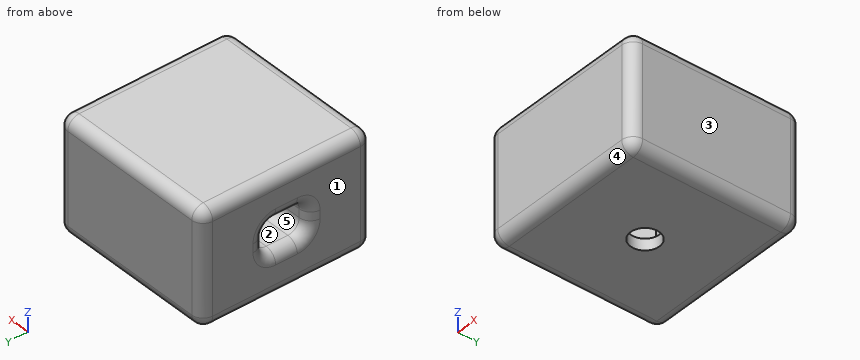
```python
from build123d import *

# Parameters (mm, degrees)
F0_W      = 38.1
F0_H      = 38.1
F1_DEPTH  = 25.4
F2_R      = 2.54
F4_DEPTH  = 33.02
F6_DEPTH  = 6.096
F7_DEPTH  = 2.54
F8_R      = 2.54
F9_R      = 3.211175
F10_DEPTH = 5.08


with BuildPart() as f1:
    # F0 (on Top) → F1 (new body)
    with BuildSketch(Plane.XY):
        Rectangle(F0_W, F0_H)
    extrude(amount=F1_DEPTH)

    # F2
    f2_edges = [f1.edges().sort_by_distance(p)[0] for p in [
        (-19.05, -19.05, 12.7),
        (-19.05, 0, 0),
        (19.05, -19.05, 12.7),
        (0, -19.05, 0),
        (0, -19.05, 25.4),
        (19.05, 0, 0),
        (0, 19.05, 0),
        (-19.05, 19.05, 12.7),
        (-19.05, 0, 25.4),
        (19.05, 0, 25.4),
        (0, 19.05, 25.4),
        (19.05, 19.05, 12.7),
    ]]
    fillet(f2_edges, radius=F2_R)

    # F3 (on face) → F4 (cut)
    with BuildSketch(Plane(origin=(-19.05, 0, 0), x_dir=(0, -1, 0), z_dir=(-1, 0, 0))):
        Polygon((4.958837, 16.184959), (0, 16.184959), (0, 12.7), (0, 9.215041), (4.958837, 9.215041), align=None)
        Polygon((0, 16.184959), (-4.958837, 16.184959), (-4.958837, 9.215041), (0, 9.215041), (0, 12.7), align=None)
    extrude(amount=-F4_DEPTH, mode=Mode.SUBTRACT)

    # F5 (on face) → F6 (cut)
    with BuildSketch(Plane(origin=(0, 0, 0), x_dir=(1, 0, 0), z_dir=(0, 0, -1))):
        Polygon((-2.712969, -4.699), (2.712969, -4.699), (5.425938, 0), (2.712969, 4.699), (-2.712969, 4.699), (-5.425938, 0), align=None)
    extrude(amount=-F6_DEPTH, mode=Mode.SUBTRACT)

    # F5 (on face) → F7 (join)
    with BuildSketch(Plane(origin=(0, 0, 0), x_dir=(1, 0, 0), z_dir=(0, 0, -1))):
        Polygon((-2.712969, -4.699), (2.712969, -4.699), (5.425938, 0), (2.712969, 4.699), (-2.712969, 4.699), (-5.425938, 0), align=None)
    extrude(amount=-F7_DEPTH)

    # F8
    f8_edges = [f1.edges().sort_by_distance(p)[0] for p in [
        (13.97, 0, 16.184959),
        (13.97, 4.958837, 12.7),
        (13.97, 0, 9.215041),
        (13.97, -4.958837, 12.7),
        (-2.54, 4.958837, 16.184959),
        (-2.54, 4.958837, 9.215041),
        (-19.05, 4.958837, 12.7),
        (-2.54, -4.958837, 16.184959),
        (-19.05, 0, 16.184959),
        (-2.54, -4.958837, 9.215041),
        (-19.05, -4.958837, 12.7),
        (-19.05, 0, 9.215041),
    ]]
    fillet(f8_edges, radius=F8_R)

    # F9 (on face) → F10 (cut)
    with BuildSketch(Plane(origin=(0, 0, 0), x_dir=(1, 0, 0), z_dir=(0, 0, -1))):
        Circle(F9_R)
    extrude(amount=-F10_DEPTH, mode=Mode.SUBTRACT)


solid = f1.part
```
Could you check a few things on this model? Use its own coordinates, in mm. Face numbers are marked on the shaded views. A direction names the side the tool comes from. Round coordinates to 2 decimals unless told otherwise and drop trailing zeros. Loops run counter-clockwise (first coordinate to the right, second up) from the corner with the lowest first, then second, coordinate; pieces in that order, holes last. Notation, with made-up numbers: (27, 56) -> (32, 56) arc R22 cw to (32, 81) -> close; hole circle Ø11 at (68, 33). An arc over 180 degrees is marked (long way). Put each result on its own line as item: value.
Q1. I want a section at B-B on x = 8. Write out the boundary of the cut face in (y, z), and give its area (3 significant figures).
Checks:
outline: (-19.05, 2.54) arc R2.54 ccw to (-16.51, 0) -> (16.51, 0) arc R2.54 ccw to (19.05, 2.54) -> (19.05, 22.86) arc R2.54 ccw to (16.51, 25.4) -> (-16.51, 25.4) arc R2.54 ccw to (-19.05, 22.86) -> close; hole (-4.96, 11.76) arc R2.54 ccw to (-2.42, 9.22) -> (2.42, 9.22) arc R2.54 ccw to (4.96, 11.76) -> (4.96, 13.64) arc R2.54 ccw to (2.42, 16.18) -> (-2.42, 16.18) arc R2.54 ccw to (-4.96, 13.64) -> close
area: 899 mm2
Q2. I want a section at A-A on x = 0. Write out the boundary of the cut face in (y, z).
Checks:
outline: (-19.05, 2.54) arc R2.54 ccw to (-16.51, 0) -> (-3.21, 0) -> (-3.21, 2.54) -> (-4.7, 2.54) -> (-4.7, 6.1) -> (4.7, 6.1) -> (4.7, 2.54) -> (3.21, 2.54) -> (3.21, 0) -> (16.51, 0) arc R2.54 ccw to (19.05, 2.54) -> (19.05, 22.86) arc R2.54 ccw to (16.51, 25.4) -> (-16.51, 25.4) arc R2.54 ccw to (-19.05, 22.86) -> close; hole (-4.96, 11.76) arc R2.54 ccw to (-2.42, 9.22) -> (2.42, 9.22) arc R2.54 ccw to (4.96, 11.76) -> (4.96, 13.64) arc R2.54 ccw to (2.42, 16.18) -> (-2.42, 16.18) arc R2.54 ccw to (-4.96, 13.64) -> close
Q3. For pin 1 Ø0.9 at (y, z) = (1, 12.5) entering from -X, with a flat end and sliding along its axis, tell me the tip position at first contact or that it passes through.
Checks:
pin 1: x = 13.97
Q4. Which directions (+Z, -Z, +X, -X, +Y, -Y) give clear straight access to the entire face, cutting with the end or side of a thin tool? Please do the marked faces 1 and 2.
Checks:
face 1: +Z, -Z, -X, +Y, -Y
face 2: -X
Q5. Thinking about a two-plate mould opening in Y: for the marked faces 3, 4 and 5, which applies, pulls with the +Y half, pulls with the -Y half, needs draft (parallel to the pull), parting line crosses it, or undercut?
Checks:
face 3: needs draft
face 4: pulls with the -Y half
face 5: undercut
Q6. Please list where these lines run through material, in increasing order: line 1 (Z direction, x = -9, y = -0.5); line 2 (Z direction, x = -11.5, y = 4.5); line 3 (Y direction, x = 0, z = 1.3). Write a range as from..to.
Checks:
line 1: 0..9.22, 16.18..25.4
line 2: 0..10.3, 15.1..25.4
line 3: -18.73..-3.21, 3.21..18.73
Q7. I want a section at C-C on y = -1.5. Write out the boundary of the cut face in (x, z).
Checks:
outline: (-19.05, 2.54) arc R2.54 ccw to (-16.51, 0) -> (-2.84, 0) -> (-2.84, 2.54) -> (-4.56, 2.54) -> (-4.56, 6.1) -> (4.56, 6.1) -> (4.56, 2.54) -> (2.84, 2.54) -> (2.84, 0) -> (16.51, 0) arc R2.54 ccw to (19.05, 2.54) -> (19.05, 22.86) arc R2.54 ccw to (16.51, 25.4) -> (-16.51, 25.4) arc R2.54 ccw to (-19.05, 22.86) -> (-19.05, 18.72) arc R2.54 ccw to (-16.51, 16.18) -> (11.43, 16.18) arc R2.54 cw to (13.97, 13.64) -> (13.97, 11.76) arc R2.54 cw to (11.43, 9.22) -> (-16.51, 9.22) arc R2.54 ccw to (-19.05, 6.68) -> close
